Geometry check sheet. Reference: the model listing, model coordinates, mm. A direction names the side the tool comes from. Round coordinates to 2 decimals unless told otherwise and drop trailing zeros. Order: outer loops, then holes, each group sorted by start corner. A loop starts at its lowest first (then second) coordinate and runs counter-clockwise, first axis right, second up.
(1) Sectioned sample at D-D (y = -19). Record the boundary of the cut face in (x, z).
(2) Sectioned sample at A-A (x = 10.5). Record the boundary of the cut face in (y, z).
(3) Sectioned sample at B-B (z = 42). Record the boundary of the cut face in (x, y).
(4) Release check for a two-part mould opening along X. For faces 4 (the face through (3.944, -36.886, 49.109)), 5 (the face through (0, -21, 62)), 6 (the face through (23, -26, 58)) record: +X half, -X half, draft (parallel to the pull), parting line (faces both ways), or undercut.
(5) Material ranges on line 1 along X through (y, z) = (-26.5, 65.5); line 2 along X through (y, z) = (-7.95, 42); line 3 along Z through (x, y) = (59.5, -10.25), recorded low to high.
(6) Sectioned sample at C-C (x = 61). Record the boundary of the cut face in (y, z), plus the area to 3 significant figures.
(7) Set-up check for faces 1 (the face through (26.451, -36.886, 49.109)), 2 (the face through (37, -46, 98.5)), 3 (the face through (37.395, -9.717, 46.308)): record each of +Z, -Z, +X, -X, +Y, -Y from which the full face is reachable in a straight line by a thin tool's end or side.
(8) Go/stop test with flat-tipped pins: pin 1 (12 mm diameter, centred on x = 66.5, z = 61, fed in from +Y); pin 2 (6 mm diameter, centred on x = 59.5, z = 17, fed in from -Y); pin 3 (8 mm diameter, centred on x = 38, y = -20.5, fed in from -Z); pin 4 (4 mm diameter, centred on x = 59.5, z = 42, fed in from +Y). Record where each tip stops, or that it passes through.
from build123d import *

# Parameters (mm, degrees)
F0_W      = 75
F0_H      = 100
F1_DEPTH  = 56
F3_DEPTH  = 75.001
F4_W      = 15
F4_H      = 92
F5_DEPTH  = 50
F6_W      = 65
F6_H      = 20
F7_DEPTH  = 1.5
F9_DEPTH  = 75.001
F11_DEPTH = 75
F12_W     = 75
F12_H     = 5
F12_R     = 2.6
F13_DEPTH = 56.001


with BuildPart() as f1:
    # F0 (on Front) → F1 (new body)
    with BuildSketch(Plane.XZ):
        with Locations((37.5, 50)):
            Rectangle(F0_W, F0_H)
    extrude(amount=F1_DEPTH)

    # F2 (on face) → F3 (cut, through all)
    with BuildSketch(Plane(origin=(0, 0, 0), x_dir=(0, -1, 0), z_dir=(-1, 0, 0))):
        Polygon((56, 92), (15, 0), (56, 0), align=None)
    extrude(amount=-F3_DEPTH, mode=Mode.SUBTRACT)

    # F4 (on face) → F5 (cut)
    with BuildSketch(Plane.XZ.offset(56)):
        with Locations((15.5, 46)):
            Rectangle(F4_W, F4_H)
        with Locations((37.5, 46)):
            Rectangle(F4_W, F4_H)
        with Locations((59.5, 46)):
            Rectangle(F4_W, F4_H)
    extrude(amount=-F5_DEPTH, mode=Mode.SUBTRACT)

    # F6 (on face) → F7 (cut)
    with BuildSketch(Plane.XY.offset(100)):
        with Locations((37.5, -46)):
            Rectangle(F6_W, F6_H)
    extrude(amount=-F7_DEPTH, mode=Mode.SUBTRACT)

    # F8 (on face) → F9 (cut, through all)
    with BuildSketch(Plane(origin=(0, 0, 0), x_dir=(0, -1, 0), z_dir=(-1, 0, 0))):
        Polygon((8.748866, 0), (0, 100), (0, 0), align=None)
    extrude(amount=-F9_DEPTH, mode=Mode.SUBTRACT)

    # F10 (on face) → F11 (join, through all)
    with BuildSketch(Plane(origin=(0, 0, 0), x_dir=(0, -1, 0), z_dir=(-1, 0, 0))):
        Polygon((5.019099, 100), (0, 100), (8.748866, 0), (13.767966, 0), align=None)
    extrude(amount=-F11_DEPTH)

    # F12 (on face) → F13 (cut, through all)
    with BuildSketch(Plane.XZ.offset(56)):
        with Locations((37.5, 2.5)):
            Rectangle(F12_W, F12_H)
        with Locations((15.5, 17)):
            Circle(F12_R)
        with Locations((15.5, 42)):
            Circle(F12_R)
        with Locations((15.5, 67)):
            Circle(F12_R)
        with Locations((37.5, 67)):
            Circle(F12_R)
        with Locations((37.5, 42)):
            Circle(F12_R)
        with Locations((37.5, 17)):
            Circle(F12_R)
        with Locations((59.5, 17)):
            Circle(F12_R)
        with Locations((59.5, 42)):
            Circle(F12_R)
        with Locations((59.5, 67)):
            Circle(F12_R)
    extrude(amount=-F13_DEPTH, mode=Mode.SUBTRACT)


solid = f1.part
Answer below:
1. outline: (0, 8.98) - (8, 8.98) - (8, 92) - (23, 92) - (23, 8.98) - (30, 8.98) - (30, 92) - (45, 92) - (45, 8.98) - (52, 8.98) - (52, 92) - (67, 92) - (67, 8.98) - (75, 8.98) - (75, 100) - (0, 100) - close
2. outline: (-56, 92) - (-6, 92) - (-6, 88.79) - (-13.33, 5) - (-8.31, 5) - (0, 100) - (-36, 100) - (-36, 98.5) - (-56, 98.5) - close
3. outline: (0, -33.72) - (8, -33.72) - (8, -10.09) - (12.9, -10.09) - (12.9, -5.07) - (0, -5.07) - close; (18.1, -10.09) - (23, -10.09) - (23, -33.72) - (30, -33.72) - (30, -10.09) - (34.9, -10.09) - (34.9, -5.07) - (18.1, -5.07) - close; (40.1, -10.09) - (45, -10.09) - (45, -33.72) - (52, -33.72) - (52, -10.09) - (56.9, -10.09) - (56.9, -5.07) - (40.1, -5.07) - close; (62.1, -10.09) - (67, -10.09) - (67, -33.72) - (75, -33.72) - (75, -5.07) - (62.1, -5.07) - close
4. face 4: draft
4. face 5: -X half
4. face 6: undercut
5. line 1: x = 0 to 8, 23 to 30, 45 to 52, 67 to 75
5. line 2: x = 0 to 12.9, 18.1 to 34.9, 40.1 to 56.9, 62.1 to 75
5. line 3: z = 5 to 14.4, 19.6 to 39.4, 92 to 100
6. outline: (-56, 92) - (-6, 92) - (-6, 88.79) - (-7.72, 69.12) - (-2.7, 69.12) - (0, 100) - (-36, 100) - (-36, 98.5) - (-56, 98.5) - close; (-13.33, 5) - (-8.31, 5) - (-7.45, 14.88) - (-12.47, 14.88) - close; (-12.09, 19.12) - (-7.08, 19.12) - (-5.26, 39.88) - (-10.28, 39.88) - close; (-9.91, 44.12) - (-4.89, 44.12) - (-3.07, 64.88) - (-8.09, 64.88) - close
6. area: 788 mm2
7. face 1: -Z, +X, -X, -Y
7. face 2: +Z, -Y
7. face 3: -Y
8. pin 1: stops at y = -2.89
8. pin 2: stops at y = -12.54
8. pin 3: stops at z = 92
8. pin 4: passes through
